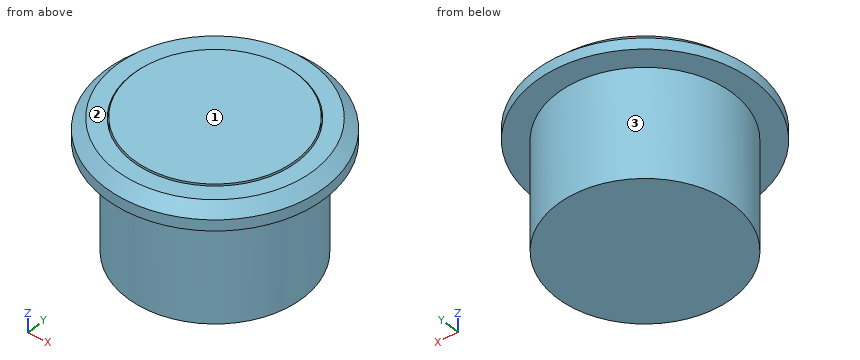
```python
from build123d import *

# Parameters (mm, degrees)
ESQUISSE1_R             = 8
BOSS_EXTRU_1_DEPTH      = 10
ESQUISSE2_R             = 10
BOSS_EXTRU_2_DEPTH      = 2
CHANFREIN1_SIZE         = 1
ESQUISSE3_R             = 7.5
ENL_V_MAT_EXTRU_1_DEPTH = 0.5
ESQUISSE4_R             = 7.4
BOSS_EXTRU_3_DEPTH      = 0.6


with BuildPart() as part:
    # Esquisse1 → Boss.-Extru.1 (new body)
    with BuildSketch(Plane.XY):
        Circle(ESQUISSE1_R)
    extrude(amount=BOSS_EXTRU_1_DEPTH)

    # Esquisse2 → Boss.-Extru.2 (add)
    with BuildSketch(Plane.XY.offset(10)):
        Circle(ESQUISSE2_R)
    extrude(amount=BOSS_EXTRU_2_DEPTH)

    # Chanfrein1
    chanfrein1_edges = [part.edges().sort_by_distance(p)[0] for p in [
        (-10, 0, 12),
    ]]
    chamfer(chanfrein1_edges, length=CHANFREIN1_SIZE)

    # Esquisse3 → Enlèv. mat.-Extru.1 (cut)
    with BuildSketch(Plane.XY.offset(12)):
        Circle(ESQUISSE3_R)
    extrude(amount=-ENL_V_MAT_EXTRU_1_DEPTH, mode=Mode.SUBTRACT)

    # Esquisse4 → Boss.-Extru.3 (add)
    with BuildSketch(Plane.XY.offset(11.5)):
        Circle(ESQUISSE4_R)
    extrude(amount=BOSS_EXTRU_3_DEPTH)


solid = part.part
```
Part model, mm, in its own coordinate system. Face numbers are marked on the shaded views. A direction names the side the tool comes from. Give positions to 0.01 mm unless a question says otherwise; leave off trailing zeros. Write each loop counter-clockwise with the first axis right and the second up, starting at its lowest first coordinate (ties: lowest second). Pieces come first, ordered by that corner, then holes. Notation, with made-up numbers: M 25,25 L 56,25 A31 cw 56,57 Z; hole C 8.25,54.5 d2. An arc over 180 degrees is marked long. Use CSV: the item, a comma, the result in double quotes.
Item 1: Slice it at C-C on z = 10.25. Write the cut outline in (x, y).
Taken from the geometry:
outline,"C 0,0 d20"
Item 2: Pin check, flat tips, straight feed: P1, Ø1.5, axis at x = -0.5, z = 5, coming from the +Y side; P2, Ø4, axis at y = -6, z = 4.5, coming from the -X side; P3, Ø5, axis at y = 7.5, z = 5.5, coming from the -X side (3 decimals). Stop position of each tip, or through.
Taken from the geometry:
P1,"stops at y = 8"
P2,"stops at x = -6.93"
P3,"stops at x = -6.245"
Item 3: Slice it at A-A on x = 0. Write the cut outline in (y, z), plus the area to 3 significant figures.
Taken from the geometry:
outline,"M -10,10 L -8,10 L -8,0 L 8,0 L 8,10 L 10,10 L 10,11 L 9,12 L 7.5,12 L 7.5,11.5 L 7.4,11.5 L 7.4,12.1 L -7.4,12.1 L -7.4,11.5 L -7.5,11.5 L -7.5,12 L -9,12 L -10,11 Z"
area,"200 mm²"
Item 4: Which spindle directions (+Z, -Z, +X, -X, +Y, -Y) get a long thin tool onto all of the face, cutting with end or side? Do the marked faces 1, 2 and 3. Say none if no direction does.
Taken from the geometry:
face 1,"+Z, +X, -X, +Y, -Y"
face 2,"+Z"
face 3,"-Z"
Item 5: Drill centre lines: probe 1 along Z at (x, y) = (7.5, 1.25); probe 2 along Y at (x, z) = (-4.25, 8.75); probe 3 along X at (y, z) = (-7.25, 3). Where is each one in solid material? Low to high.
Taken from the geometry:
probe 1,"z = 0 to 12"
probe 2,"y = -6.78 to 6.78"
probe 3,"x = -3.38 to 3.38"
Item 6: Slice it at D-D on z = 7.5. Write the cut outline in (x, y), plus the area to 3 significant figures.
Taken from the geometry:
outline,"C 0,0 d16"
area,"201 mm²"
